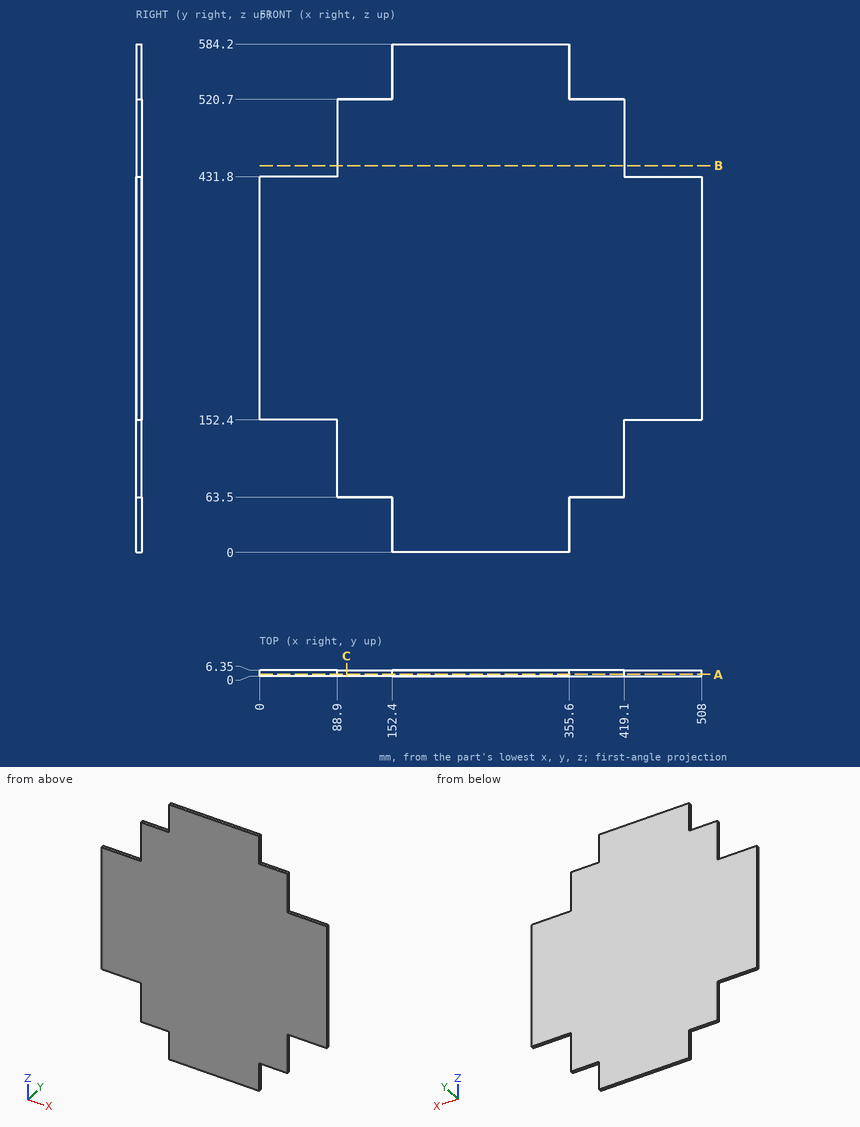
Could you check a few things on this drawing? It's one solid part, dimensions in mm from its lowest x, y, z. Give positions to 0.01 mm unless a question says otherwise; leave off trailing zeros. Write each loop counter-clockwise with the first axis right and the second up, starting at its lowest first coordinate (ties: lowest second). Pieces come first, ordered by that corner, then holes.
(1) If I drill on L1, parallel to Z at x = 45.5, y = 4.25; L2, parallel to X at y = 5, z = 502; L3, parallel to X at y = 0.75, z = 545, over which ranges is the centre line in solid material (lowest first)?
Output values:
L1: z = 152.4 to 431.8
L2: x = 88.9 to 419.1
L3: x = 152.4 to 355.6
(2) Will these pins go through, and if not, where does the flat tip stop? pin 1 (1.9 mm diameter, centred on x = 121, y = 4.5, fed in from -Z); pin 2 (3 mm diameter, centred on y = 3, z = 26, fed in from +X); pin 3 (3 mm diameter, centred on x = 479, y = 4.5, fed in from +Z).
Output values:
pin 1: stops at z = 63.5
pin 2: stops at x = 355.6
pin 3: stops at z = 431.8
(3) Imagine slicing it at A-A, the plane y = 2. Write out the boundary of the cut face in (x, z), and give its area (3 significant figures).
Output values:
outline: (0, 152.4) - (88.9, 152.4) - (88.9, 63.5) - (152.4, 63.5) - (152.4, 0) - (355.6, 0) - (355.6, 63.5) - (419.1, 63.5) - (419.1, 152.4) - (508, 152.4) - (508, 431.8) - (419.1, 431.8) - (419.1, 520.7) - (355.6, 520.7) - (355.6, 584.2) - (152.4, 584.2) - (152.4, 520.7) - (88.9, 520.7) - (88.9, 431.8) - (0, 431.8) - close
area: 226,000 mm2
(4) Imagine slicing it at C-C, the plane x = 100. Write out the boundary of the cut face in (y, z).
Output values:
outline: (0, 63.5) - (6.35, 63.5) - (6.35, 520.7) - (0, 520.7) - close
(5) Imagine slicing it at B-B, the plane z = 444.5. Write out the boundary of the cut face in (x, y).
Output values:
outline: (88.9, 0) - (419.1, 0) - (419.1, 6.35) - (88.9, 6.35) - close
